Check sheet for the modelled part. Datum: model origin and axes. Units: mm. Face numbers are marked on the shaded views. A direction names the side the tool comes from. Give positions to 0.01 mm unless a question says otherwise; leave off trailing zeros. Write each loop counter-clockwise with the first axis right and the second up, starting at its lowest first coordinate (ties: lowest second). Pieces come first, ordered by that corner, then holes. Notation, with made-up numbers: M 35.5,-40 L 49.5,-40 A19 cw 49.5,-11 Z; hole C 39.25,23 d4. An arc over 180 degrees is marked long. Write item = value, one per line. Start each with the question number.
1) Sectioned sample at A-A, the plane x = 0. Record the cut outline in (y, z).
2) Sectioned sample at D-D, the plane z = -4.5. Record the cut outline in (x, y).
3) Draft check along Z on the marked faces 3, 4 and 5. Enter one of: pulls with the +Z half, pulls with the -Z half, needs draft (parallel to the pull), parting line crosses it, or undercut.
4) Set-up check for the marked faces 1 and 2: record each of +Z, -Z, +X, -X, +Y, -Y from which the full face is reachable in a straight line by a thin tool's end or side.
5) Gauge pin test, flat ends, axial feed: pin 1 (3 mm diameter, centred on y = 9, z = 2, fed in from +X); pin 2 (3 mm diameter, centred on x = -4.5, y = 13.5, fed in from -Z); pin 3 (5 mm diameter, centred on x = -4, y = 14.5, fed in from -Z). Record the tip position at first contact, or that the pin passes through.
6) Sectioned sample at C-C, the plane y = 8.5. Record the cut outline in (x, z), then the cut area to 3 significant figures.
7) Sectioned sample at B-B, the plane z = 0.5. Record the cut outline in (x, y).
8) Scan lines: L1, parallel to Z at x = 0, y = 4.25; L2, parallel to X at y = 21.5, z = 0. Record each from-to range of solid material in increasing order.
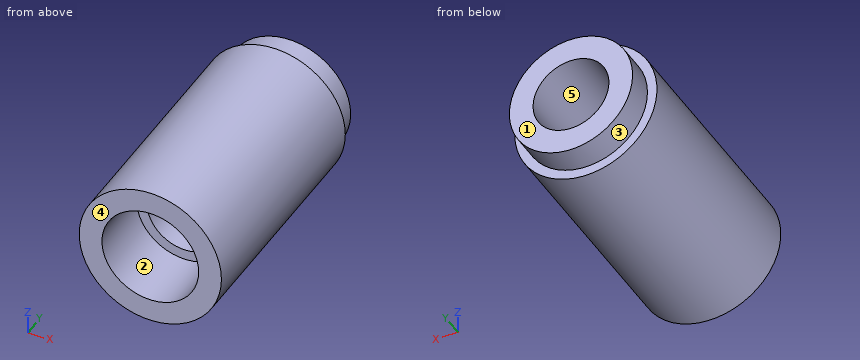
from build123d import *

# Parameters (mm, degrees)
SKETCH1_R           = 7.5
BOSS_EXTRUDE1_DEPTH = 25
SKETCH2_R           = 6.5
BOSS_EXTRUDE2_DEPTH = 3
SKETCH3_R           = 5.1
CUT_EXTRUDE1_DEPTH  = 7
SKETCH4_R           = 4
CUT_EXTRUDE2_DEPTH  = 29


with BuildPart() as part:
    # Sketch1 → Boss-Extrude1 (new body)
    with BuildSketch(Plane(origin=(0, 0, 0), x_dir=(1, 0, 0), z_dir=(0, 1, 0))):
        Circle(SKETCH1_R)
    extrude(amount=BOSS_EXTRUDE1_DEPTH)

    # Sketch2 → Boss-Extrude2 (add)
    with BuildSketch(Plane(origin=(0, 25, 0), x_dir=(1, 0, 0), z_dir=(0, 1, 0))):
        Circle(SKETCH2_R)
    extrude(amount=BOSS_EXTRUDE2_DEPTH)

    # Sketch3 → Cut-Extrude1 (cut)
    with BuildSketch(Plane.XZ):
        Circle(SKETCH3_R)
    extrude(amount=-CUT_EXTRUDE1_DEPTH, mode=Mode.SUBTRACT)

    # Sketch4 → Cut-Extrude2 (cut, through all)
    with BuildSketch(Plane(origin=(0, 28, 0), x_dir=(1, 0, 0), z_dir=(0, 1, 0))):
        Circle(SKETCH4_R)
    extrude(amount=-CUT_EXTRUDE2_DEPTH, mode=Mode.SUBTRACT)


solid = part.part
Data:
q1.outline = M 0,-7.5 L 25,-7.5 L 25,-6.5 L 28,-6.5 L 28,-4 L 7,-4 L 7,-5.1 L 0,-5.1 Z; M 0,5.1 L 7,5.1 L 7,4 L 28,4 L 28,6.5 L 25,6.5 L 25,7.5 L 0,7.5 Z
q2.outline = M -6,0 L -2.4,0 L -2.4,7 L 2.4,7 L 2.4,0 L 6,0 L 6,25 L 4.69,25 L 4.69,28 L -4.69,28 L -4.69,25 L -6,25 Z
q3.face_3 = parting line crosses it
q3.face_4 = needs draft
q3.face_5 = undercut
q4.face_1 = +Z, -Z, +X, -X, +Y
q4.face_2 = -Y
q5.pin_1 = 7.48
q5.pin_2 = -6.87
q5.pin_3 = -7.35
q6.outline = C 0,0 d15; hole C 0,0 d8
q6.area = 126 mm2
q7.outline = M -7.48,0 L -5.08,0 L -5.08,7 L -3.97,7 L -3.97,28 L -6.48,28 L -6.48,25 L -7.48,25 Z; M 3.97,7 L 5.08,7 L 5.08,0 L 7.48,0 L 7.48,25 L 6.48,25 L 6.48,28 L 3.97,28 Z
q8.L1 = -7.5 to -5.1, 5.1 to 7.5
q8.L2 = -7.5 to -4, 4 to 7.5
